Check sheet for the modelled part. Datum: model origin and axes. Units: mm. Face numbers are marked on the shaded views. A direction names the side the tool comes from. Give positions to 0.01 mm unless a question says otherwise; leave off trailing zeros. Write each loop counter-clockwise with the first axis right and the second up, starting at its lowest first coordinate (ties: lowest second). Pieces come first, ordered by that corner, then holes.
Autodesk Inventor part; units mm, degrees
ref_plane "YZ Plane" through (0, 0, 0) normal (1, 0, 0) x (0, 1, 0)
ref_plane "XZ Plane" through (0, 0, 0) normal (0, 1, 0) x (-1, 0, 0)
ref_plane "XY Plane" through (0, 0, 0) normal (0, 0, 1) x (1, 0, 0)
sketch "Sketch1" plane through (0, 0, 0) normal (0, 0, 1) x (1, 0, 0)
  line L0 (0, 0) -> (11.9253, 0)
  line L1 (11.9253, 0) -> (11.9253, 9.9314)
  line L2 (11.9253, 9.9314) -> (0, 9.9314)
  line L3 (0, 9.9314) -> (0, 0)
  dimension "d0" = 11.9253
  dimension "d1" = 9.9314
extrude "Extrusion1" add sketch "Sketch1" along normal blind 8.89
sketch "Sketch2" plane through (0, 0, 8.89) normal (0, 0, 1) x (1, 0, 0)
  circle A0 centre (5.9626, 4.9657) radius 1.5
  line L0 (11.9253, 9.9314) -> (0, 9.9314) construction
  line L1 (0, 9.9314) -> (0, 0) construction
  point P0 (5.9626, 9.9314)
  point P1 (0, 4.9657)
  dimension "d4" = 3
extrude "Extrusion2" add sketch "Sketch2" along normal blind 10.16
sketch "Sketch3" plane through (0, 0, 8.89) normal (0, 0, 1) x (1, 0, 0)
  circle A0 centre (10.4711, 4.9657) radius 0.762
  circle A1 centre (1.4541, 4.9657) radius 0.762
  line L0 (1.4541, 4.9657) -> (0, 4.9657) construction
  line L1 (0, 9.9314) -> (0, 0) construction
  line L2 (10.4711, 4.9657) -> (11.9253, 4.9657) construction
  line L3 (11.9253, 0) -> (11.9253, 9.9314) construction
  dimension "d7" = 9.017
  dimension "d8" = 1.524
extrude "Extrusion3" cut sketch "Sketch3" against normal blind 7.62
sketch "Sketch4" plane through (0, 0, 0) normal (0, 0, -1) x (-1, 0, 0)
  line L0 (0, 0) -> (-11.9253, 0) construction
  line L1 (0, 9.9314) -> (0, 0) construction
  line L2 (-11.9253, 9.9314) -> (0, 9.9314) construction
  line L3 (-11.9253, 0) -> (-11.9253, 9.9314) construction
  line L4 (-11.9253, 9.9314) -> (0, 9.9314)
  line L5 (-1.8351, 9.9314) -> (-10.0901, 9.9314)
  line L6 (0, 0) -> (-11.9253, 0)
  line L7 (-1.8351, 0) -> (-10.0901, 0)
  arc A0 (-10.0901, 9.9314) -> (-10.0901, 0) centre (-4.2894, 4.9657) ccw
  arc A1 (-1.8351, 0) -> (-1.8351, 9.9314) centre (-7.6359, 4.9657) ccw
  line L8 (0, 9.9314) -> (0, 0)
  line L9 (-11.9253, 0) -> (-11.9253, 9.9314)
  dimension "d11" = 8.255
extrude "Extrusion4" add sketch "Sketch4" along normal blind 15.24 contours L4 A1 L6 A0
sketch "Sketch5" plane through (0, 0, -15.24) normal (0, 0, -1) x (-1, 0, 0)
  circle A0 centre (-5.9626, 4.9657) radius 1.5 construction
  circle A1 centre (-5.9626, 4.9657) radius 1.5
  circle A2 centre (-5.9626, 4.9657) radius 2.2225
  point P0 (0, 0)
  dimension "d14" = 4.445
extrude "Extrusion5" add sketch "Sketch5" along normal blind 1.27 contours A1 | A2
properties part number "MicroGearMotor" material "Brass, Soft Yellow, Welded"
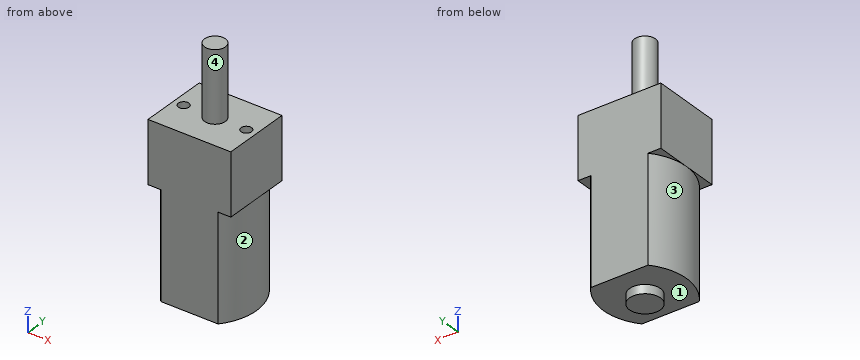
1) Scan lines: L1, parallel to X at y = 5, z = 4; L2, parallel to Z at x = 8.5, y = 9.5; L3, parallel to Z at x = 11.5, y = 1.5. Record each from-to range of solid material in increasing order.
2) Access from +Z, -Z, +X, -X, +Y, -Y to the whole of each face (thin tool, end or side, straight path). Record for the marked faces 1, 2, 3 and 4.
3) Sectioned sample at D-D on x = 2.75. Record the boundary of the cut face in (y, z).
4) Sectioned sample at B-B on y = 7.5. Record the boundary of the cut face in (x, z), then the cut area to 3 significant figures.
5) Gauge pin test, flat ends, axial feed: pin 1 (2 mm diameter, centred on x = 1.45, y = 4.97, fed in from -Z); pin 2 (3 mm diameter, centred on x = 7, y = 7, fed in from +Z); pin 3 (1 mm diameter, centred on x = 10, y = 2.5, fed in from +Z); pin 4 (6 mm diameter, centred on x = 9, z = 12.5, fed in from -Y). Record the tip position at first contact, or that the pin passes through.
6) Sectioned sample at C-C on z = 11. Record the boundary of the cut face in (x, y), then the cut area to 3 significant figures.
7) Sectioned sample at A-A on z = 2.5. Record the boundary of the cut face in (x, y), then the cut area to 3 significant figures.
Answers below:
1. L1: x = 0 to 0.69, 2.22 to 9.71, 11.23 to 11.93
1. L2: z = -15.24 to 8.89
1. L3: z = 0 to 8.89
2. face 1: -Z
2. face 2: -Z, +X
2. face 3: -Z, -X
2. face 4: +Z
3. outline: (0, -15.24) - (9.93, -15.24) - (9.93, 8.89) - (0, 8.89) - close
4. outline: (0, 0) - (0.43, 0) - (0.43, -15.24) - (11.49, -15.24) - (11.49, 0) - (11.93, 0) - (11.93, 8.89) - (0, 8.89) - close
4. area: 275 mm2
5. pin 1: stops at z = -15.24
5. pin 2: stops at z = 19.05
5. pin 3: stops at z = 8.89
5. pin 4: stops at y = 3.47
6. outline: circle Ø3 at (5.96, 4.97)
6. area: 7.07 mm2
7. outline: (0, 0) - (11.93, 0) - (11.93, 9.93) - (0, 9.93) - close; hole circle Ø1.52 at (1.45, 4.97); hole circle Ø1.52 at (10.47, 4.97)
7. area: 115 mm2
